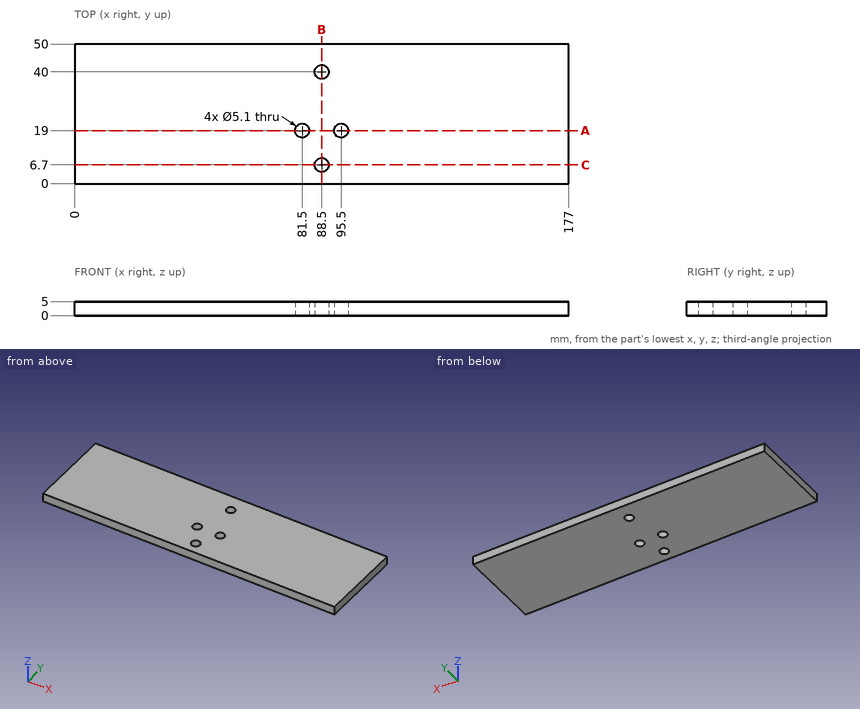
Could you check a few things on this drawing? It's one solid part, dimensions in mm from its lowest x, y, z. Give positions to 0.01 mm unless a question says otherwise; leave off trailing zeros. Order: outer loops, then holes, each group sorted by start corner. A loop starts at its lowest first (then second) coordinate and runs counter-clockwise, first axis right, second up. Notation, with made-up numbers: (40, 8) -> (90, 8) arc R22 ccw to (90, 19) -> close; hole circle Ø1 at (-8.75, 30). An arc over 180 degrees is marked (long way). Use CSV: the item, a comma, the result in double quotes. Start each with the question number.
Item 1: Suppose I cut it at A-A (y = 19). List the corners of the cut face in (x, z) for me.
Item 2: Suppose I cut it at B-B (x = 88.5). List the corners of the cut face in (y, z) for me.
Item 3: Suppose I cut it at C-C (y = 6.7). List the corners of the cut face in (x, z) for me.
Item 4: If I drill on probe 1 along Y at (x, z) = (88.5, 1.7); probe 2 along Y at (x, z) = (95.5, 1.3); probe 3 along X at (y, z) = (20.5, 4.7), over which ranges is the centre line in solid material (lowest first)? Write a range as [from, to].
Item 5: I'm going to push a flat-ended pin straight in: P1, Ø4, axis at x = 81.5, y = 19, coming from the -Z side. Where does the tip first touch, or does it pass through?
Answer block:
1,outline,"(0, 0) -> (78.95, 0) -> (78.95, 5) -> (0, 5) -> close; (84.05, 0) -> (92.95, 0) -> (92.95, 5) -> (84.05, 5) -> close; (98.05, 0) -> (177, 0) -> (177, 5) -> (98.05, 5) -> close"
2,outline,"(0, 0) -> (4.15, 0) -> (4.15, 5) -> (0, 5) -> close; (9.25, 0) -> (37.45, 0) -> (37.45, 5) -> (9.25, 5) -> close; (42.55, 0) -> (50, 0) -> (50, 5) -> (42.55, 5) -> close"
3,outline,"(0, 0) -> (85.95, 0) -> (85.95, 5) -> (0, 5) -> close; (91.05, 0) -> (177, 0) -> (177, 5) -> (91.05, 5) -> close"
4,probe 1,"y = [0, 4.15], [9.25, 37.45], [42.55, 50]"
4,probe 2,"y = [0, 16.45], [21.55, 50]"
4,probe 3,"x = [0, 79.44], [83.56, 93.44], [97.56, 177]"
5,P1,"passes through"
